Verification items for this drawing (mm, ordinates from the low corner). A direction names the side the tool comes from. Coordinates: 2 decimals unless noted, no trailing zeros. Order: outer loops, then holes, each group sorted by start corner. A loop starts at its lowest first (then second) coordinate and runs counter-clockwise, first axis right, second up. Notation, with made-up numbers: (84.25, 44.25) - (117.25, 44.25) arc R10 cw to (117.25, 56.25) - close; hole circle Ø2 at (47, 14.5). An arc over 180 degrees is marked (long way). Use CSV: the item, a comma, the result in double quotes. Start each with the question number.
1) Sectioned sample at D-D, the plane x = 5.25. Record the cut outline in (y, z).
2) Thickness scan on probe 1 along Y at (x, z) = (9, 1.05); probe 2 along Z at (x, y) = (9.5, 30). Record the ranges inside material, lowest first. Write a range as [from, to].
3) Depth check by flat-ended pin: P1, Ø4, axis at x = 11.5, y = 29.5, coming from the -Z side; P2, Ø3.5, axis at x = 9.5, y = 24.5, coming from the +Z side; P3, Ø3.5, axis at y = 23.5, z = 19.9, coming from the +X side; P4, Ø2, axis at y = 35.5, z = 6, coming from the +X side. Enter the tip coordinate at first touch or a pass-through.
4) Sectioned sample at A-A, the plane x = 9. Record the cut outline in (y, z).
5) Sectioned sample at B-B, the plane y = 23.5. Record the cut outline in (x, z).
6) Tool access check on the marked faces 1 and 2. Record the directions out of +Z, -Z, +X, -X, +Y, -Y that give a thin tool (end or side, any length) a straight path to the whole face; none if there is none.
7) Sectioned sample at C-C, the plane z = 20.5. Record the cut outline in (x, y).
8) Draft check along Y on the marked faces 3, 4, 5 and 6. Enter one of: released by +Y, released by -Y, zero draft, split by the parting line, or undercut.
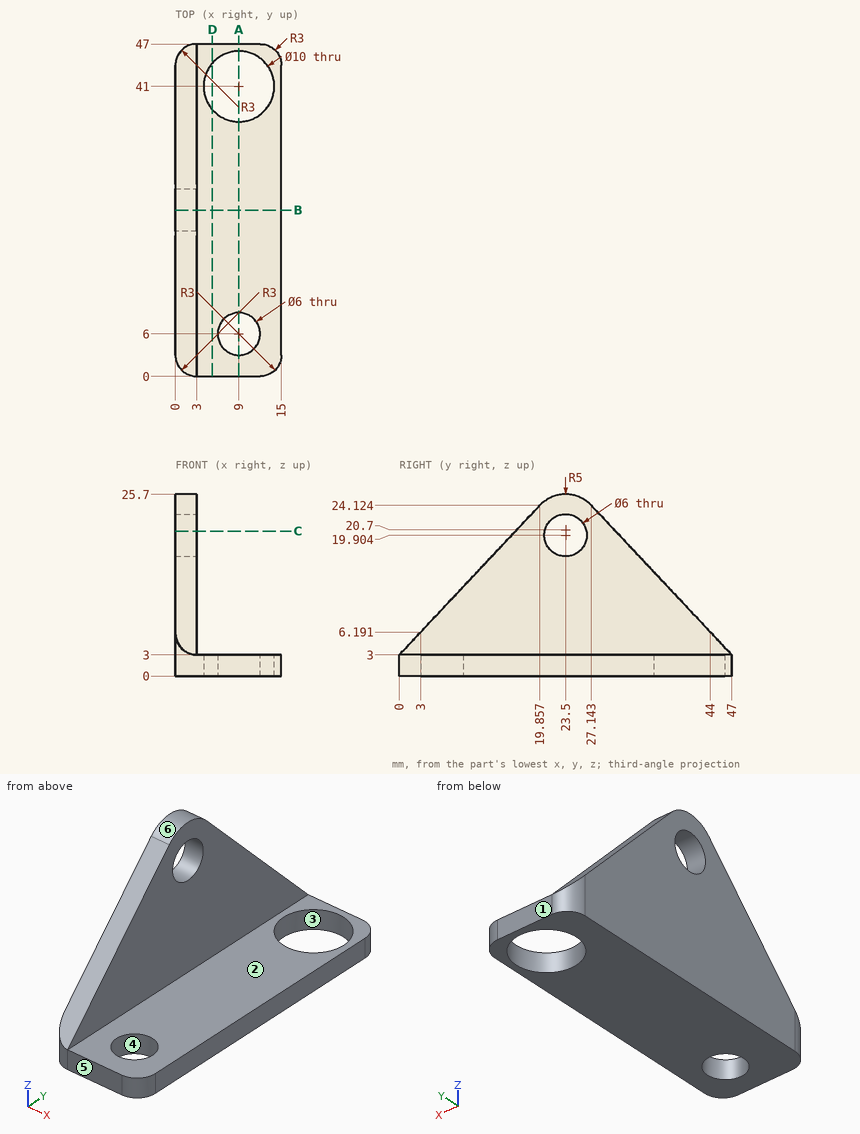
Evaluation:
1,outline,"(0, 0) - (37.69, 0) - (37.69, 3) - (0, 3) - close; (44.31, 0) - (47, 0) - (47, 3) - (44.31, 3) - close"
2,probe 1,"[0, 3], [9, 36], [46, 47]"
2,probe 2,"[0, 3]"
3,P1,"z = 0"
3,P2,"z = 3"
3,P3,"through"
3,P4,"x = 3"
4,outline,"(0, 0) - (3, 0) - (3, 3) - (0, 3) - close; (9, 0) - (36, 0) - (36, 3) - (9, 3) - close; (46, 0) - (47, 0) - (47, 3) - (46, 3) - close"
5,outline,"(0, 0) - (15, 0) - (15, 3) - (3, 3) - (3, 16.9) - (0, 16.9) - close; (0, 22.9) - (3, 22.9) - (3, 25.7) - (0, 25.7) - close"
6,face 1,"+Z, -Z, +X, -X, +Y"
6,face 2,"+Z, +X, +Y, -Y"
7,outline,"(0, 16.45) - (3, 16.45) - (3, 20.56) - (0, 20.56) - close; (0, 26.44) - (3, 26.44) - (3, 30.55) - (0, 30.55) - close"
8,face 3,"undercut"
8,face 4,"undercut"
8,face 5,"released by -Y"
8,face 6,"split by the parting line"
